from build123d import *

# Parameters (mm, degrees)
F1_DEPTH = 15
F3_D     = 9.5
F5_D     = 3.2
F5_DEPTH = 7.5
F5_TIP   = 0.9613769904
F6_R     = 5


with BuildPart() as f1:
    # F0 (on Top) → F1 (new body)
    with BuildSketch(Plane.XY):
        Polygon((-38, 0), (0, 0), (0, -28), (12, -28), (12, 12), (-38, 12), align=None)
    extrude(amount=-F1_DEPTH)

    # F3 (through all)
    with Locations(Plane.XZ):
        with Locations((-31, -7.5)):
            Hole(F3_D / 2)

    # F5
    with Locations(Plane.XY):
        with Locations((-31, 6)):
            Hole(F5_D / 2, depth=F5_DEPTH)
            with Locations((0, 0, -(F5_DEPTH + F5_TIP / 2))):  # 118° drill point
                Cone(0, F5_D / 2, F5_TIP, mode=Mode.SUBTRACT)

    # F6
    f6_edges = [f1.edges().sort_by_distance(p)[0] for p in [
        (0, 0, -7.5),
    ]]
    fillet(f6_edges, radius=F6_R)


solid = f1.part
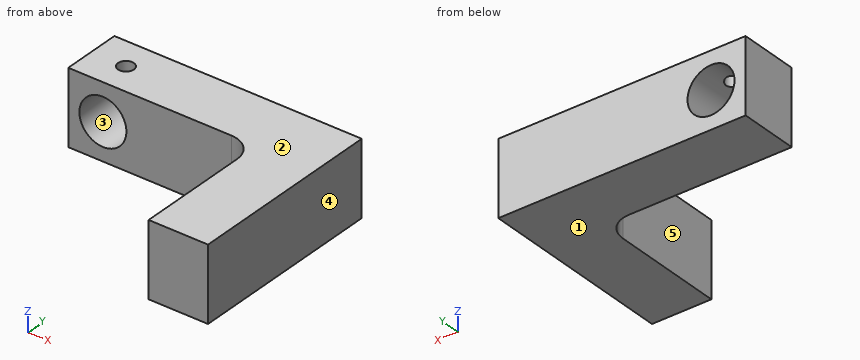
Work out the finished part from the listing and answer in its coordinate system (mm). Face numbers are marked on the shaded views. A direction names the side the tool comes from. Round coordinates to 2 decimals unless told otherwise and drop trailing zeros. Loops run counter-clockwise (first coordinate to the right, second up) from the corner with the lowest first, then second, coordinate; pieces in that order, holes last. Notation, with made-up numbers: (-3, -22.75) - (43, -22.75) arc R10 cw to (43, -17.75) - close; hole circle Ø4 at (63.25, 8.25). An arc over 180 degrees is marked (long way). One line per item, written item: value.
Q1. Each of these flat-tipped pins is pushed along its axis until it touches: pin 1 Ø3 at (x, y) = (-31, 6) entering from +Z; pin 2 Ø7.5 at (x, z) = (-13.5, -5) entering from -Y; pin 3 Ø2 at (y, z) = (-15.5, -13) entering from -X. Where does it stop, or does it pass through?
Check values:
pin 1: z = -12.01
pin 2: y = 0
pin 3: x = 0
Q2. Find section C-C on y = 6. Give the vertices of the cut face in (x, z).
Check values:
outline: (-38, -15) - (12, -15) - (12, 0) - (-29.4, 0) - (-29.4, -3.03) arc R4.75 cw (long way) to (-32.6, -3.03) - (-32.6, 0) - (-38, 0) - close
Q3. The mould has two halves that part along Z. Classify the marked faces 1, 2 and 3: +Z half, -Z half, draft (parallel to the pull), parting line (faces both ways), or undercut.
Check values:
face 1: -Z half
face 2: +Z half
face 3: undercut
Q4. Find section D-D on x = -16. Give the vertices of the cut face in (y, z), and give its area (3 significant figures).
Check values:
outline: (0, -15) - (12, -15) - (12, 0) - (0, 0) - close
area: 180 mm2
Q5. For the marked faces 4 and 5, determine the directions among +Z, -Z, +X, -X, +Y, -Y from which every point of the face is accessible in a straight line to the end or side of a thin tool.
Check values:
face 4: +Z, -Z, +X, +Y, -Y
face 5: +Z, -Z, -X, -Y
Q6. Straight lines are drawn through the part: probe 1 along Z at (x, y) = (-31, 9); probe 2 along X at (y, z) = (-8, -13); probe 3 along Y at (x, z) = (-31, -1.5). For each, find the intervals that lie inside material, in ascending order.
Check values:
probe 1: -15 to -12.25, -2.75 to 0
probe 2: 0 to 12
probe 3: 0 to 4.4, 7.6 to 12
Q7. Find section A-A on z = -7.5. Give the vertices of the cut face in (x, y).
Check values:
outline: (-38, 0) - (-35.75, 0) - (-35.75, 12) - (-38, 12) - close; (-26.25, 0) - (-5, 0) arc R5 cw to (0, -5) - (0, -28) - (12, -28) - (12, 12) - (-26.25, 12) - close
Q8. Find section B-B on x = -31. Give the vertices of the cut face in (y, z), and give its area (3 significant figures).
Check values:
outline: (0, -15) - (12, -15) - (12, -12.25) - (0, -12.25) - close; (0, -2.75) - (4.4, -2.75) - (4.4, 0) - (0, 0) - close; (7.6, -2.75) - (12, -2.75) - (12, 0) - (7.6, 0) - close
area: 57.2 mm2
